from build123d import *

# Parameters (mm, degrees)
SKETCH1_W               = 42
SKETCH1_H               = 42
BOSS_EXTRUDE4_DEPTH     = 10
CUT_EXTRUDE3_DEPTH      = 117.726175299
CUT_EXTRUDE3_DEPTH_BACK = 4
SKETCH5_W               = 17
SKETCH5_H               = 10
BOSS_EXTRUDE5_DEPTH     = 10
CUT_EXTRUDE5_DEPTH      = 119.004237212
CUT_EXTRUDE5_DEPTH_BACK = 119.004237212
SKETCH8_W               = 10
SKETCH8_H               = 10
BOSS_EXTRUDE6_DEPTH     = 15
BOSS_EXTRUDE7_START     = -10.28
SKETCH10_W              = 42
SKETCH10_H              = 42
SKETCH10_W_2            = 38
SKETCH10_H_2            = 38
BOSS_EXTRUDE7_DEPTH     = 2
BOSS_EXTRUDE8_START     = -10
SKETCH11_W              = 42
SKETCH11_H              = 42
SKETCH11_W_2            = 38
SKETCH11_H_2            = 38
BOSS_EXTRUDE8_DEPTH     = 2
SKETCH12_W              = 5
SKETCH12_H              = 7.5
SKETCH12_H_2            = 6
SKETCH12_W_2            = 23
SKETCH12_H_3            = 23
SKETCH12_W_3            = 19
SKETCH12_H_4            = 19
SKETCH12_H_5            = 2
SKETCH12_W_4            = 7.5
SKETCH12_H_6            = 3
SKETCH12_W_5            = 2
BOSS_EXTRUDE9_DEPTH     = 2
SKETCH15_W              = 5
SKETCH15_H              = 2
BOSS_EXTRUDE12_DEPTH    = 1.72
SKETCH16_W              = 3
SKETCH16_H              = 2
BOSS_EXTRUDE13_DEPTH    = 2
SKETCH17_W              = 3
SKETCH17_H              = 2
BOSS_EXTRUDE14_DEPTH    = 2
SKETCH19_W              = 19
SKETCH19_H              = 8
BOSS_EXTRUDE15_DEPTH    = 2
SKETCH20_W              = 19
SKETCH20_H              = 19
CUT_EXTRUDE6_DEPTH      = 2
SKETCH21_W              = 5
SKETCH21_H              = 2
BOSS_EXTRUDE16_DEPTH    = 2


with BuildPart() as part:
    # Sketch1 → Boss-Extrude4 (new body)
    with BuildSketch(Plane(origin=(0, 0, 0), x_dir=(1, 0, 0), z_dir=(0, 1, 0))):
        Polygon((-25, -25), (25, -25), (55, -25), (105, -25), (105, 25), (55, 25), (25, 25), (-25, 25), align=None)
        with Locations((80, 0)):
            Rectangle(SKETCH1_W, SKETCH1_H, mode=Mode.SUBTRACT)
        Rectangle(SKETCH1_W, SKETCH1_H, mode=Mode.SUBTRACT)
    extrude(amount=BOSS_EXTRUDE4_DEPTH)

    # Sketch5 → Cut-Extrude3 (cut, two sides: drawn at the far end of the back side and taken through both)
    with BuildSketch(Plane.XY.offset(25).offset(-CUT_EXTRUDE3_DEPTH_BACK)):
        with Locations((0, 5)):
            Rectangle(SKETCH5_W, SKETCH5_H)
        with Locations((80, 5)):
            Rectangle(SKETCH5_W, SKETCH5_H)
    extrude(amount=CUT_EXTRUDE3_DEPTH + CUT_EXTRUDE3_DEPTH_BACK, mode=Mode.SUBTRACT)

    # Sketch6 → Boss-Extrude5 (add)
    with BuildSketch(Plane(origin=(0, 10, 0), x_dir=(1, 0, 0), z_dir=(0, 1, 0))):
        Polygon((105, 25), (40, 25), (40, -25), (71.5, -25), (71.5, -21), (59, -21), (59, 21), (101, 21), (101, -21), (88.5, -21), (88.5, -25), (105, -25), align=None)
    extrude(amount=BOSS_EXTRUDE5_DEPTH)

    # Sketch8 → Cut-Extrude5 (cut, two sides: drawn at the far end of the back side and taken through both)
    with BuildSketch(Plane.XY.offset(25).offset(-CUT_EXTRUDE5_DEPTH_BACK)):
        with Locations((45, 15)):
            Rectangle(SKETCH8_W, SKETCH8_H)
    extrude(amount=CUT_EXTRUDE5_DEPTH + CUT_EXTRUDE5_DEPTH_BACK, mode=Mode.SUBTRACT)

    # Sketch9 → Boss-Extrude6 (add)
    with BuildSketch(Plane.XZ):
        Polygon((-21, 21), (-8.5, 21), (-8.5, 25), (-25, 25), (-25, -25), (105, -25), (105, 25), (88.5, 25), (88.5, 21), (101, 21), (101, -21), (59, -21), (59, 21), (71.5, 21), (71.5, 25), (8.5, 25), (8.5, 21), (21, 21), (21, -21), (-21, -21), align=None)
    extrude(amount=BOSS_EXTRUDE6_DEPTH)

    # Sketch10 → Boss-Extrude7 (add)
    with BuildSketch(Plane(origin=(0, 10, 0), x_dir=(1, 0, 0), z_dir=(0, 1, 0)).offset(BOSS_EXTRUDE7_START)):
        Rectangle(SKETCH10_W, SKETCH10_H)
        Rectangle(SKETCH10_W_2, SKETCH10_H_2, mode=Mode.SUBTRACT)
    extrude(amount=-BOSS_EXTRUDE7_DEPTH)

    # Sketch11 → Boss-Extrude8 (add)
    with BuildSketch(Plane(origin=(0, 20, 0), x_dir=(1, 0, 0), z_dir=(0, 1, 0)).offset(BOSS_EXTRUDE8_START)):
        with Locations((80, 0)):
            Rectangle(SKETCH11_W, SKETCH11_H)
        with Locations((80, 0)):
            Rectangle(SKETCH11_W_2, SKETCH11_H_2, mode=Mode.SUBTRACT)
    extrude(amount=-BOSS_EXTRUDE8_DEPTH)

    # Sketch12 → Boss-Extrude9 (add)
    # profile 1 of 10: a face of its own
    with BuildSketch(Plane(origin=(0, -4, 0), x_dir=(1, 0, 0), z_dir=(0, 1, 0))):
        with Locations((0, 15.25)):
            Rectangle(SKETCH12_W, SKETCH12_H)
    # profile 2 of 10: a face of its own
    with BuildSketch(Plane(origin=(0, -4, 0), x_dir=(1, 0, 0), z_dir=(0, 1, 0))):
        with Locations((0, 22)):
            Rectangle(SKETCH12_W, SKETCH12_H_2)
    # profile 3 of 10: a face of its own
    with BuildSketch(Plane(origin=(0, -4, 0), x_dir=(1, 0, 0), z_dir=(0, 1, 0))):
        Rectangle(SKETCH12_W_2, SKETCH12_H_3)
        Rectangle(SKETCH12_W_3, SKETCH12_H_4, mode=Mode.SUBTRACT)
    # profile 4 of 10: a face of its own
    with BuildSketch(Plane(origin=(0, -4, 0), x_dir=(1, 0, 0), z_dir=(0, 1, 0))):
        with Locations((0, -15.25)):
            Rectangle(SKETCH12_W, SKETCH12_H)
    # profile 5 of 10: a face of its own
    with BuildSketch(Plane(origin=(0, -4, 0), x_dir=(1, 0, 0), z_dir=(0, 1, 0))):
        with Locations((0, -20)):
            Rectangle(SKETCH12_W, SKETCH12_H_5)
    # profile 6 of 10: a face of its own
    with BuildSketch(Plane(origin=(0, -4, 0), x_dir=(1, 0, 0), z_dir=(0, 1, 0))):
        with Locations((-15.25, 0)):
            Rectangle(SKETCH12_W_4, SKETCH12_H_6)
    # profile 7 of 10: a face of its own
    with BuildSketch(Plane(origin=(0, -4, 0), x_dir=(1, 0, 0), z_dir=(0, 1, 0))):
        with Locations((-10.5, 0)):
            Rectangle(SKETCH12_W_5, SKETCH12_H_6)
    # profile 8 of 10: a face of its own
    with BuildSketch(Plane(origin=(0, -4, 0), x_dir=(1, 0, 0), z_dir=(0, 1, 0))):
        Polygon((-9.5, -1.5), (-11.5, -1.5), (-11.5, -11.5), (-2.5, -11.5), (2.5, -11.5), (11.5, -11.5), (11.5, -1.5), (9.5, -1.5), (9.5, -9.5), (2.5, -9.5), (-2.5, -9.5), (-9.5, -9.5), align=None)
    # profile 9 of 10: a face of its own
    with BuildSketch(Plane(origin=(0, -4, 0), x_dir=(1, 0, 0), z_dir=(0, 1, 0))):
        with Locations((10.5, 0)):
            Rectangle(SKETCH12_W_5, SKETCH12_H_6)
    # profile 10 of 10: a face of its own
    with BuildSketch(Plane(origin=(0, -4, 0), x_dir=(1, 0, 0), z_dir=(0, 1, 0))):
        with Locations((15.25, 0)):
            Rectangle(SKETCH12_W_4, SKETCH12_H_6)
    extrude(amount=-BOSS_EXTRUDE9_DEPTH)

    # Sketch15 → Boss-Extrude12 (add)
    with BuildSketch(Plane(origin=(0, -4, 0), x_dir=(1, 0, 0), z_dir=(0, 1, 0))):
        with Locations((0, -20)):
            Rectangle(SKETCH15_W, SKETCH15_H)
    extrude(amount=BOSS_EXTRUDE12_DEPTH)

    # Sketch16 → Boss-Extrude13 (add)
    with BuildSketch(Plane.ZY.offset(19)):
        with Locations((0, -5)):
            Rectangle(SKETCH16_W, SKETCH16_H)
    extrude(amount=BOSS_EXTRUDE13_DEPTH)

    # Sketch17 → Boss-Extrude14 (add)
    with BuildSketch(Plane(origin=(19, 0, 0), x_dir=(0, 0, -1), z_dir=(1, 0, 0))):
        with Locations((0, -5)):
            Rectangle(SKETCH17_W, SKETCH17_H)
    extrude(amount=BOSS_EXTRUDE14_DEPTH)

    # Sketch19 → Boss-Extrude15 (add)
    with BuildSketch(Plane(origin=(0, 6.28, 0), x_dir=(1, 0, 0), z_dir=(0, 1, 0))):
        Polygon((91.5, 11.5), (82.5, 11.5), (82.5, 21), (77.5, 21), (77.5, 11.5), (68.5, 11.5), (68.5, 1.5), (59, 1.5), (59, -1.5), (68.5, -1.5), (68.5, -11.5), (77.5, -11.5), (77.5, -21), (82.5, -21), (82.5, -11.5), (91.5, -11.5), (91.5, -1.5), (101, -1.5), (101, 1.5), (91.5, 1.5), align=None)
        with Locations((80, -5.5)):
            Rectangle(SKETCH19_W, SKETCH19_H, mode=Mode.SUBTRACT)
        with Locations((80, 5.5)):
            Rectangle(SKETCH19_W, SKETCH19_H, mode=Mode.SUBTRACT)
    extrude(amount=-BOSS_EXTRUDE15_DEPTH)

    # Sketch20 → Cut-Extrude6 (cut)
    with BuildSketch(Plane(origin=(0, 6.28, 0), x_dir=(1, 0, 0), z_dir=(0, 1, 0))):
        with Locations((80, 0)):
            Rectangle(SKETCH20_W, SKETCH20_H)
    extrude(amount=-CUT_EXTRUDE6_DEPTH, mode=Mode.SUBTRACT)

    # Sketch21 → Boss-Extrude16 (add)
    with BuildSketch(Plane(origin=(0, 6.28, 0), x_dir=(1, 0, 0), z_dir=(0, 1, 0))):
        with Locations((80, -20)):
            Rectangle(SKETCH21_W, SKETCH21_H)
    extrude(amount=BOSS_EXTRUDE16_DEPTH)


solid = part.part
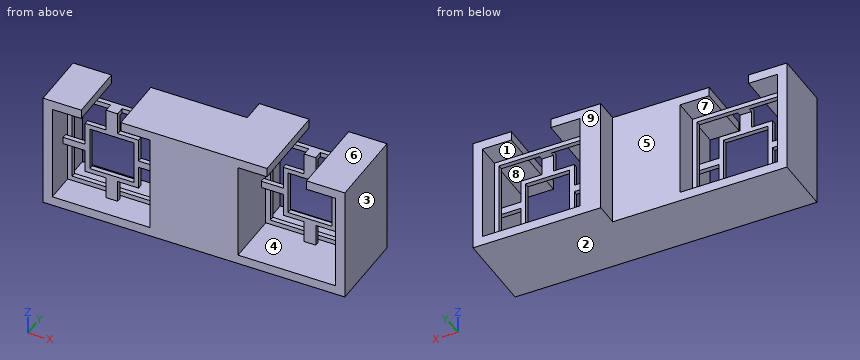
The model under review builds one solid part; all positions refer to its coordinate system, in mm. Face numbers are marked on the shaded views. A direction names the side the tool comes from. Round coordinates to 2 decimals unless told otherwise and drop trailing zeros. Loops run counter-clockwise (first coordinate to the right, second up) from the corner with the lowest first, then second, coordinate; pieces in that order, holes last. Notation, with made-up numbers: (49, 27.25) -> (57, 27.25) arc R8 cw to (57, 39.25) -> close; hole circle Ø5 at (-4, 89.5). An arc over 180 degrees is marked (long way). Write item = value, one per line. Start each with the question number.
Item 1: For the marked faces 5, 6, 7, 8 and 9, list the 3-axis set-ups (+Z, -Z, +X, -X, +Y, -Y) from which the entire face can be reached by the end or side of a thin tool; tool diameter is ignored.
Item 2: Mouldability with a two-part tool opening along X and no side actions: class the marked faces 1, 2, 3 and 4 as released by +X, released by -X, zero draft, split by the parting line, or undercut.
Item 3: Insertion check: pin 1 (0.6 mm diameter, centred on x = 73, y = 5, fed in from +Z); pin 2 (7 mm diameter, centred on x = 84, y = 2, fed in from +Z); pin 3 (1 mm diameter, centred on x = -11.5, z = 4, fed in from -Y). Each pin has a flat end and moves straight along its axis. Give the tip position at first contact, or say it passes through.
Item 4: Take a section at B-B on y = 15.5. Give the boundary of the cut face in (x, z).
Item 5: To check wall thickness, follow L1, parallel to X at y = -5, z = -19.5; L2, parallel to X at y = -11.5, z = 10; L3, parallel to X at y = 16.5, z = 20. State the ranges of each line that lie inside material, in increasing order.
Item 6: Take a section at C-C on z = -14.5. Count the separate pieces of the cut face and the enclosed holes in it, plus the area to 3 significant figures.
Item 7: Take a section at A-A on x = -7. Give the boundary of the cut face in (y, z).
Result:
q1.face_5 = +Z, -Z, -X, +Y
q1.face_6 = +Z, +X, -X, +Y, -Y
q1.face_7 = +Y
q1.face_8 = -Y
q1.face_9 = +Z, -Z, +X, -X, +Y
q2.face_1 = undercut
q2.face_2 = zero draft
q2.face_3 = released by +X
q2.face_4 = undercut
q3.pin_1 = 11.5
q3.pin_2 = 21
q3.pin_3 = -6
q4.outline = (50, -25) -> (105, -25) -> (105, 25) -> (88.5, 25) -> (88.5, 21) -> (101, 21) -> (101, -21) -> (59, -21) -> (59, 21) -> (71.5, 21) -> (71.5, 25) -> (50, 25) -> close
q5.L1 = -25 to -21, -2.5 to 2.5, 21 to 59, 101 to 105
q5.L2 = -25 to -21, 21 to 59, 101 to 105
q5.L3 = 50 to 59, 101 to 105
q6.separate_pieces = 5
q6.enclosed_holes = 0
q6.area = 1,320 mm²
q7.outline = (-15, -25) -> (10, -25) -> (10, -21) -> (-0.28, -21) -> (-0.28, -19) -> (-2.28, -19) -> (-2.28, -21) -> (-15, -21) -> close; (-6, -11.5) -> (-4, -11.5) -> (-4, -9.5) -> (-6, -9.5) -> close; (-6, 9.5) -> (-4, 9.5) -> (-4, 11.5) -> (-6, 11.5) -> close; (-2.28, 19) -> (-0.28, 19) -> (-0.28, 21) -> (-2.28, 21) -> close
